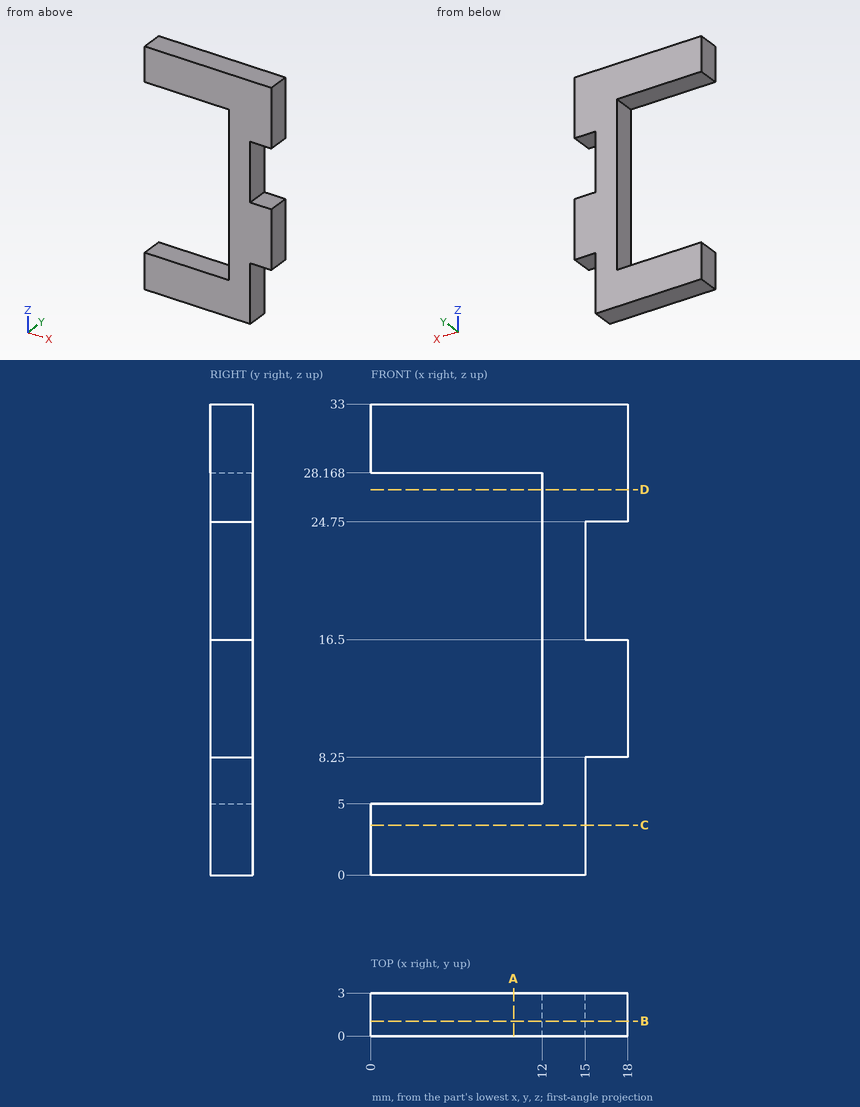
Check sheet for the drawn part. Datum: minimum x, y, z corner. Units: mm. Round coordinates to 2 decimals unless told otherwise and drop trailing zeros. Write each loop counter-clockwise with the first axis right and the second up, starting at its lowest first coordinate (ties: lowest second). Pieces come first, ordered by that corner, then holes. Notation, with made-up numbers: (63.5, -29.75) -> (69.5, -29.75) arc R10 cw to (69.5, -12.75) -> close; hole circle Ø5 at (46, -4.5). An arc over 180 degrees is marked (long way). Write each question's results on one line, items separated by ' | '.
Q1. Sectioned sample at A-A, the plane x = 10. Record the boundary of the cut face in (y, z).
Derived:
outline: (0, 0) -> (3, 0) -> (3, 5) -> (0, 5) -> close; (0, 28.17) -> (3, 28.17) -> (3, 33) -> (0, 33) -> close
Q2. Sectioned sample at D-D, the plane z = 27. Record the boundary of the cut face in (x, y).
Derived:
outline: (12, 0) -> (18, 0) -> (18, 3) -> (12, 3) -> close
Q3. Sectioned sample at C-C, the plane z = 3.5. Record the boundary of the cut face in (x, y), and give its area (3 significant figures).
Derived:
outline: (0, 0) -> (15, 0) -> (15, 3) -> (0, 3) -> close | area: 45.0 mm²
Q4. Thickness scan on probe 1 along Z at (x, y) = (10, 1.45); probe 2 along Z at (x, y) = (17.25, 1.1); probe 3 along X at (y, z) = (2.8, 10). Record the ranges inside material, lowest first.
Derived:
probe 1: z = 0 to 5, 28.17 to 33 | probe 2: z = 8.25 to 16.5, 24.75 to 33 | probe 3: x = 12 to 18
Q5. Sectioned sample at B-B, the plane y = 1.05. Record the boundary of the cut face in (x, z).
Derived:
outline: (0, 0) -> (15, 0) -> (15, 8.25) -> (18, 8.25) -> (18, 16.5) -> (15, 16.5) -> (15, 24.75) -> (18, 24.75) -> (18, 33) -> (0, 33) -> (0, 28.17) -> (12, 28.17) -> (12, 5) -> (0, 5) -> close
Q6. Go/stop test with flat-tipped pins: pin 1 Ø1 at (x, y) = (6.5, 1.5) entering from -Z; pin 2 Ø1.5 at (x, y) = (16.5, 2) entering from -Z. Record where each tip stops, or that it passes through.
Derived:
pin 1: stops at z = 0 | pin 2: stops at z = 8.25
